```python
from build123d import *

# Parameters (mm, degrees)
F0_W      = 19.5
F0_H      = 6
F1_DEPTH  = 0.5
F2_R      = 1.25
F3_DEPTH  = 3
F4_W      = 11.4
F4_H      = 2
F5_DEPTH  = 0.2
F6_W      = 1.5
F6_H      = 2
F7_DEPTH  = 4.7
F8_W      = 11.5
F8_H      = 6
F9_DEPTH  = 5.2
F10_W     = 1.6
F10_H     = 6
F11_DEPTH = 2.4
F12_R     = 0.4
F13_DEPTH = 6


with BuildPart() as f1:
    # F0 (on Front) → F1 (new body)
    with BuildSketch(Plane.XZ):
        with Locations((9.75, -3)):
            Rectangle(F0_W, F0_H)
    extrude(amount=F1_DEPTH)

    # F2 (on face) → F3 (cut)
    with BuildSketch(Plane.XZ.offset(0.5)):
        with Locations((2, -3)):
            Circle(F2_R)
        with Locations((17, -3)):
            Circle(F2_R)
    extrude(amount=-F3_DEPTH, mode=Mode.SUBTRACT)

    # F4 (on face) → F5 (cut)
    with BuildSketch(Plane.XZ.offset(0.5)):
        with Locations((9.7, -2.875332)):
            Rectangle(F4_W, F4_H)
    extrude(amount=-F5_DEPTH, mode=Mode.SUBTRACT)

    # F6 (on face) → F7 (join)
    with BuildSketch(Plane.XZ.offset(0.3)):
        with Locations((13.65, -2.875332)):
            Rectangle(F6_W, F6_H)
    extrude(amount=F7_DEPTH)

    # F8 (on face) → F9 (join)
    with BuildSketch(Plane(origin=(0, 0, 0), x_dir=(-1, 0, 0), z_dir=(0, 1, 0))):
        with Locations((-9.5, -3)):
            Rectangle(F8_W, F8_H)
    extrude(amount=F9_DEPTH)

    # F10 (on face) → F11 (join)
    with BuildSketch(Plane(origin=(0, 5.2, 0), x_dir=(-1, 0, 0), z_dir=(0, 1, 0))):
        with Locations((-12.95, -3)):
            Rectangle(F10_W, F10_H)
        with Locations((-9.5, -3)):
            Rectangle(F10_W, F10_H)
        with Locations((-6.05, -3)):
            Rectangle(F10_W, F10_H)
    extrude(amount=F11_DEPTH)

    # F12 (on face) → F13 (cut)
    with BuildSketch(Plane.XY):
        with Locations((12.95, 7)):
            Circle(F12_R)
        with Locations((9.5, 7)):
            Circle(F12_R)
        with Locations((6.05, 7)):
            Circle(F12_R)
    extrude(amount=-F13_DEPTH, mode=Mode.SUBTRACT)


solid = f1.part
```
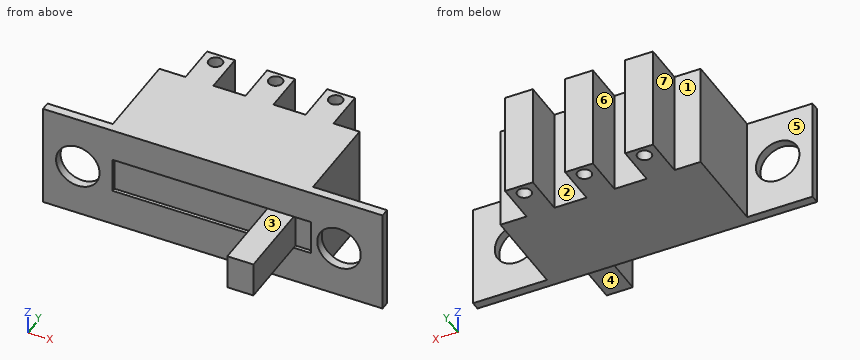
The model under review builds one solid part; all positions refer to its coordinate system, in mm. Face numbers are marked on the shaded views. A direction names the side the tool comes from. Round coordinates to 2 decimals unless told otherwise and drop trailing zeros. Order: outer loops, then holes, each group sorted by start corner. A loop starts at its lowest first (then second) coordinate and runs counter-clockwise, first axis right, second up. Notation, with made-up numbers: M -8.75,-18.75 L 27.25,-18.75 A15 ccw 27.25,-11.75 Z; hole C 76.25,32 d3. An arc over 180 degrees is marked long. Use a Markdown table: item, result.
1) Consider section B-B (z = -1.5). Write out the cut boundary in (x, y).
Report:
| item | result |
|---|---|
| outline | M 0,-0.5 L 19.5,-0.5 L 19.5,0 L 15.25,0 L 15.25,5.2 L 13.75,5.2 L 13.75,7.6 L 12.15,7.6 L 12.15,5.2 L 10.3,5.2 L 10.3,7.6 L 8.7,7.6 L 8.7,5.2 L 6.85,5.2 L 6.85,7.6 L 5.25,7.6 L 5.25,5.2 L 3.75,5.2 L 3.75,0 L 0,0 Z; hole C 6.05,7 d0.8; hole C 9.5,7 d0.8; hole C 12.95,7 d0.8 |
2) Draft analysis for pull direction X (two halves, no side actions). For the marked faces 5, 6 and 7, state which applies: released by +X, released by -X, zero draft, split by the parting line, or undercut.
Report:
| item | result |
|---|---|
| face 5 | zero draft |
| face 6 | undercut |
| face 7 | released by -X |
3) Consider section A-A (x = 18). Write out the cut boundary in (y, z).
Report:
| item | result |
|---|---|
| outline | M -0.5,-6 L 0,-6 L 0,-3.75 L -0.5,-3.75 Z; M -0.5,-2.25 L 0,-2.25 L 0,0 L -0.5,0 Z |
4) Consider section D-D (y = -2). Write out the cut boundary in (x, z).
Report:
| item | result |
|---|---|
| outline | M 12.9,-3.88 L 14.4,-3.88 L 14.4,-1.88 L 12.9,-1.88 Z |
5) Wall thickness on line 1 along X through (y, z) = (6, -4.4); line 2 along Y through (x, z) = (12.95, -2); line 3 along Z through (x, y) = (17, -0.25): over which ranges is each line inside the solid? List them lowest first. Write a range as [from, to].
Report:
| item | result |
|---|---|
| line 1 | [5.25, 6.85], [8.7, 10.3], [12.15, 13.75] |
| line 2 | [-5, 6.6], [7.4, 7.6] |
| line 3 | [-6, -4.25], [-1.75, 0] |
6) Insertion check: pin 1 (0.8 mm diameter, centred on x = 13.5, y = -3.5, fed in from +Z); pin 2 (0.7 mm diameter, centred on y = 7, z = -1.5, fed in from +X); pin 3 (2.5 mm diameter, centred on y = 3.5, z = -3, fed in from +X). Each pin has a flat end and moves straight along its axis. Give the tip position at first contact, or say it passes through.
Report:
| item | result |
|---|---|
| pin 1 | z = -1.88 |
| pin 2 | x = 13.75 |
| pin 3 | x = 15.25 |
7) Consider section C-C (x = 7.75). Write out the cut boundary in (y, z), then the cut area to 3 significant figures.
Report:
| item | result |
|---|---|
| outline | M -0.5,-6 L 5.2,-6 L 5.2,0 L -0.5,0 L -0.5,-1.88 L -0.3,-1.88 L -0.3,-3.88 L -0.5,-3.88 Z |
| area | 33.8 mm^2 |
8) Tool access review of the marked faces 1, 2, 3 and 4: name each direction out of +Z, -Z, +X, -X, +Y, -Y from which nothing blocks a thin tool from reaching the whole face with its end or side.
Report:
| item | result |
|---|---|
| face 1 | +Z, -Z, -X, +Y |
| face 2 | +Z, -Z, +Y |
| face 3 | +Z, +X, -X, -Y |
| face 4 | -Z, +X, -X, -Y |
